from build123d import *

# Parameters (mm, degrees)
F1_DEPTH  = 25
F3_DEPTH  = 130
F4_DEPTH  = 25
F5_R      = 5
F7_DEPTH  = 130
F8_DEPTH  = 25
F9_R      = 5
F10_R     = 1
F11_W     = 100
F11_H     = 10
F12_DEPTH = 35
F13_W     = 100
F13_H     = 8.0795794725
F14_DEPTH = 35
F15_R     = 5
F16_R     = 1


with BuildPart() as f1:
    # F0 (on Front) → F1 (new body)
    with BuildSketch(Plane.XZ):
        with BuildLine():
            ThreePointArc((-57.7942286341, 13.5), (-53.9433654568, 17.090109324), (-48.7430907909, 17.9118))
            Line((-48.7430907909, 17.9118), (50.034012295, 3.9804))
            ThreePointArc((50.034012295, 3.9804), (51.2644385711, 3.3117495349), (51.7546991374, 2))
            Line((51.7546991374, 2), (51.7546991374, 0.25))
            Line((51.7546991374, 0.25), (59.7546991374, 0.25))
            Line((59.7546991374, 0.25), (59.7546991374, 27))
            Line((59.7546991374, 27), (-80.5, 27))
            Line((-80.5, 27), (-80.5, 1))
            Line((-80.5, 1), (-72.5, 1))
            Line((-72.5, 1), (-72.5, 13.5))
            Line((-72.5, 13.5), (-57.7942286341, 13.5))
        make_face()
    extrude(amount=F1_DEPTH)

    # F2 (on face) → F3 (join)
    with BuildSketch(Plane(origin=(-80.5, 0, 0), x_dir=(0, -1, 0), z_dir=(-1, 0, 0))):
        Polygon((0, 1), (0, 27), (0, 35), (-10, 35), (-10, 1), align=None)
    extrude(amount=-F3_DEPTH)

    # F4 (cut): a face of the model
    f4_faces = [f1.faces().sort_by_distance(p)[0] for p in [
        (-23.2155862484, 0, 7.0978499246),
    ]]
    extrude(f4_faces, amount=-F4_DEPTH, mode=Mode.SUBTRACT)

    # F5
    f5_edges = [f1.edges().sort_by_distance(p)[0] for p in [
        (49.5, 0, 15.527858),
    ]]
    fillet(f5_edges, radius=F5_R)

    # F6 (on face) → F7 (join)
    with BuildSketch(Plane(origin=(-80.5, 0, 0), x_dir=(0, -1, 0), z_dir=(-1, 0, 0))):
        Polygon((25, 35), (25, 27), (25, 1), (33.0795794725, 1), (33.0795794725, 35), align=None)
    extrude(amount=-F7_DEPTH)

    # F8 (cut): a face of the model
    f8_faces = [f1.faces().sort_by_distance(p)[0] for p in [
        (-23.2155862484, -25, 7.0978499246),
    ]]
    extrude(f8_faces, amount=-F8_DEPTH, mode=Mode.SUBTRACT)

    # F9
    f9_edges = [f1.edges().sort_by_distance(p)[0] for p in [
        (49.5, -25, 15.527858),
    ]]
    fillet(f9_edges, radius=F9_R)

    # F10
    f10_edges = [f1.edges().sort_by_distance(p)[0] for p in [
        (-72.5, -11.53979, 13.5),
    ]]
    fillet(f10_edges, radius=F10_R)

    # F11 (on face) → F12 (cut)
    with BuildSketch(Plane.XY.offset(35)):
        with Locations((-15.5, 5)):
            Rectangle(F11_W, F11_H)
    extrude(amount=-F12_DEPTH, mode=Mode.SUBTRACT)

    # F13 (on face) → F14 (cut)
    with BuildSketch(Plane.XY.offset(35)):
        with Locations((-15.5, -29.0397897363)):
            Rectangle(F13_W, F13_H)
    extrude(amount=-F14_DEPTH, mode=Mode.SUBTRACT)

    # F15
    f15_edges = [f1.edges().sort_by_distance(p)[0] for p in [
        (-65.5, -25, 20.25),
        (-65.5, 0, 20.25),
        (34.5, 0, 16.585649),
        (34.5, -25, 16.585649),
    ]]
    fillet(f15_edges, radius=F15_R)

    # F16
    f16_edges = [f1.edges().sort_by_distance(p)[0] for p in [
        (42, -25, 27),
        (-73, -25, 27),
        (-73, 0, 27),
        (42, 0, 27),
    ]]
    fillet(f16_edges, radius=F16_R)


solid = f1.part
Model file for the job. Use its own axes, mm. A direction names the side the tool comes from. Give positions to 0.01 mm unless a question says otherwise; leave off trailing zeros. Order: outer loops, then holes, each group sorted by start corner. A loop starts at its lowest first (then second) coordinate and runs counter-clockwise, first axis right, second up. Notation, with made-up numbers: M 80.25,54.5 L 125.25,54.5 A11 cw 125.25,58.5 Z; hole C 68,-14 d9. An arc over 180 degrees is marked long. Write item = value, one per line.
Q1. Cut at A-A, the plane z = 32. List the corners of the cut face in (x, y), then the cut area to 3 significant figures.
Derived:
outline = M -80.5,-33.08 L -65.5,-33.08 L -65.5,-25 L -80.5,-25 Z; M -80.5,0 L -65.5,0 L -65.5,10 L -80.5,10 Z; M 34.5,-33.08 L 49.5,-33.08 L 49.5,-25 L 34.5,-25 Z; M 34.5,0 L 49.5,0 L 49.5,10 L 34.5,10 Z
area = 542 mm2
Q2. Flat gauge pins, fed straight in: pin 1 (2 mm diameter, centred on x = -33, y = -6.5, fed in from +Z); pin 2 (9 mm diameter, centred on y = 5.5, z = 23.5, fed in from +X); pin 3 (4 mm diameter, centred on x = 56, z = 12, fed in from +Y); pin 4 (10 mm diameter, centred on x = 43, y = -4.5, fed in from +Z). Where does each tip first touch, or does it go through?
Derived:
pin_1 = 27
pin_2 = 51.5
pin_3 = 0.03
pin_4 = 35
Q3. Drill centre lines: line 1 (Y direction, x = 47.5, z = 28); line 2 (Y direction, x = -38, z = 25.5); line 3 (X direction, y = 6.5, z = 21). Where is each one in solid material? Low to high. Write a range as [from, to].
Derived:
line_1 = [-33.08, -25], [0, 10]
line_2 = [-25, 0]
line_3 = [-80.5, -65.5], [34.5, 49.5]
Q4. Cut at C-C, the plane z = 9. List the corners of the cut face in (x, y), then the cut area to 3 significant figures.
Derived:
outline = M -80.5,-33.08 L -72.5,-33.08 L -72.5,10 L -80.5,10 Z; M 14.44,-25 L 29.5,-25 A5 cw 34.5,-30 L 34.5,-33.08 L 49.5,-33.08 L 49.5,-30 A5 cw 54.5,-25 L 59.75,-25 L 59.75,0 L 54.5,0 A5 cw 49.5,5 L 49.5,10 L 34.5,10 L 34.5,5 A5 cw 29.5,0 L 14.44,0 Z
area = 1,770 mm2
Q5. Two-plate mould, pull along Y, no slides. Class faces 4 (the cylindrical face through (33, 1.43, 16.44)), 5 (the flat face through (-72.5, -11, 7)), 6 (the flat face through (-9, -12, 27)): pulls with the +Y half, pulls with the -Y half, needs draft (parallel to the pull), parting line crosses it, or undercut.
Derived:
face_4 = pulls with the +Y half
face_5 = needs draft
face_6 = undercut
Q6. Cut at B-B, the plane y = -14. List the corners of the cut face in (x, z).
Derived:
outline = M -80.5,1 L -72.5,1 L -72.5,12.5 A1 cw -71.5,13.5 L -57.79,13.5 A9 cw -48.74,17.91 L 50.03,3.98 A2 cw 51.75,2 L 51.75,0.25 L 59.75,0.25 L 59.75,27 L -80.5,27 Z
Q7. Tool access for faces 1 (the flat face through (42, -25, 32)), 2 (the flat face through (-77, -11, 1)), 3 (the flat face through (-0.046, -11.238, 11.044)): list every direction of +Z, -Z, +X, -X, +Y, -Y with a clear straight run to the whole face (end or side of a thin tool).
Derived:
face_1 = +Z, +X, -X
face_2 = -Z, -X, +Y, -Y
face_3 = -Z, +Y, -Y
Q8. Cut at D-D, the plane x = 48. List the corners of the cut face in (y, z), then the cut area to 3 significant figures.
Derived:
outline = M -33.08,4.27 L 10,4.27 L 10,35 L 0,35 L 0,28 A1 cw -1,27 L -24,27 A1 cw -25,28 L -25,35 L -33.08,35 Z
area = 1,120 mm2
